Build history of the part. All positions in model axes, mm. Face numbers are marked on the shaded views. A direction names the side the tool comes from. Round coordinates to 2 decimals unless told otherwise and drop trailing zeros. Loops run counter-clockwise (first coordinate to the right, second up) from the corner with the lowest first, then second, coordinate; pieces in that order, holes last.
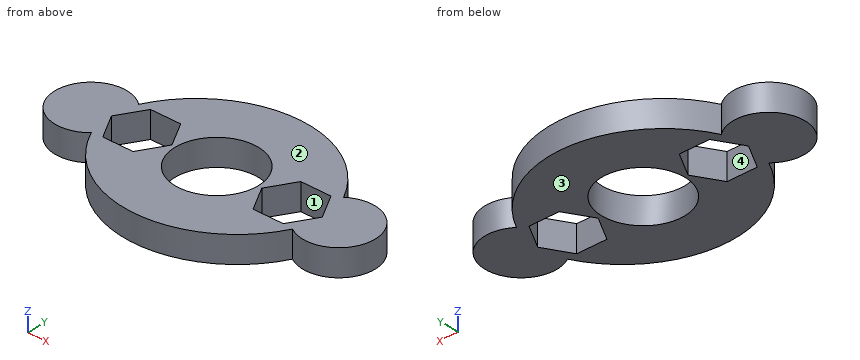
from build123d import *

# Parameters (mm, degrees)
F0_R     = 10.95
F1_DEPTH = 7


with BuildPart() as f1:
    # F0 (on Top) → F1 (new body)
    with BuildSketch(Plane.XY):
        with BuildLine():
            ThreePointArc((26.886002, -7.262236), (28.368444, -3.711389), (29.384189, 0))
            ThreePointArc((29.384189, 0), (28.162244, 4.291398), (26.317312, 8.35409))
            ThreePointArc((26.317312, 8.35409), (-0.849322, 23.940708), (-27.090225, 6.841477))
            ThreePointArc((-27.090225, 6.841477), (-28.443651, 3.48996), (-29.384189, 0))
            ThreePointArc((-29.384189, 0), (-28.351909, -3.759326), (-26.840855, -7.35305))
            ThreePointArc((-26.840855, -7.35305), (0.050708, -23.95269), (26.886002, -7.262236))
        make_face()
        Polygon((-28.139647, 0), (-24.098195, 7), (-16.015291, 7), (-11.973839, 0), (-16.015291, -7), (-24.098195, -7), align=None, mode=Mode.SUBTRACT)
        Circle(F0_R, mode=Mode.SUBTRACT)
        Polygon((28.21831, 0), (24.176858, -7), (16.093955, -7), (12.052503, 0), (16.093955, 7), (24.176858, 7), align=None, mode=Mode.SUBTRACT)
        with BuildLine():
            ThreePointArc((-29.384189, 0), (-28.443651, 3.48996), (-27.090225, 6.841477))
            ThreePointArc((-27.090225, 6.841477), (-42.77684, -0.53356), (-26.840855, -7.35305))
            ThreePointArc((-26.840855, -7.35305), (-28.351909, -3.759326), (-29.384189, 0))
        make_face()
        with BuildLine():
            ThreePointArc((26.317312, 8.35409), (28.162244, 4.291398), (29.384189, 0))
            ThreePointArc((29.384189, 0), (28.368444, -3.711389), (26.886002, -7.262236))
            ThreePointArc((26.886002, -7.262236), (41.495648, 1.088313), (26.317312, 8.35409))
        make_face()
    extrude(amount=F1_DEPTH)


solid = f1.part
(1) Pin check, flat tips, straight feed: P1, Ø4, axis at y = -10, z = 6, coming from the -X side; P2, Ø1.5, axis at y = 3, z = 2, coming from the -X side; P3, Ø1.5, axis at x = -13, z = 2.5, coming from the +Y side. Stop position of each tip, or through.
Responses:
P1: stops at x = -38.93
P2: stops at x = -42.41
P3: stops at y = 21.34
(2) Pull direction X, two halves, no side cores. Call the marked faces 1 and 2: +X half, -X half, draft (parallel to the pull), parting line (faces both ways), or undercut.
Responses:
face 1: undercut
face 2: draft
(3) Which spindle directions (+Z, -Z, +X, -X, +Y, -Y) get a long thin tool onto all of the face, cutting with end or side? Do the marked faces 3 and 4. Say none if no direction does.
Responses:
face 3: -Z, +X, -X, +Y, -Y
face 4: +Z, -Z
(4) Slice it at D-D on z = 2.25. List the corners of the cut face in (x, y), plus the area to 3 significant figures.
Responses:
outline: (-27.09, 6.84) arc R9.5 ccw (long way) to (-26.84, -7.35) arc R30 ccw to (26.89, -7.26) arc R9.5 ccw (long way) to (26.32, 8.35) arc R30 ccw to start; hole (-28.14, 0) - (-24.1, -7) - (-16.02, -7) - (-11.97, 0) - (-16.02, 7) - (-24.1, 7) - close; hole circle Ø21.9 at (0, 0); hole (12.05, 0) - (16.09, -7) - (24.18, -7) - (28.22, 0) - (24.18, 7) - (16.09, 7) - close
area: 1,840 mm2
(5) Slice it at B-B on y = -1.5. List the corners of the cut face in (x, z).
Responses:
outline: (-42.71, 0) - (-27.27, 0) - (-27.27, 7) - (-42.71, 7) - close; (-12.84, 0) - (-10.85, 0) - (-10.85, 7) - (-12.84, 7) - close; (10.85, 0) - (12.92, 0) - (12.92, 7) - (10.85, 7) - close; (27.35, 0) - (41.23, 0) - (41.23, 7) - (27.35, 7) - close
(6) Probe line 1 (Y direction, x = 0, z = 4.25); line 2 (Y direction, x = 0.5, z = 6); line 3 (X direction, y = -3.5, z = 3.5). List the from-to ranges inside material, lowest first.
Responses:
line 1: y = -23.95 to -10.95, 10.95 to 23.95
line 2: y = -23.95 to -10.94, 10.94 to 23.95
line 3: x = -42.25 to -26.12, -13.99 to -10.38, 10.38 to 14.07, 26.2 to 40.5
(7) Slice it at C-C on x = -19. List the corners of the cut face in (y, z).
Responses:
outline: (-17.17, 0) - (-7, 0) - (-7, 7) - (-17.17, 7) - close; (7, 0) - (17.17, 0) - (17.17, 7) - (7, 7) - close
(8) Slice it at A-A on x = 0. List the corners of the cut face in (y, z), plus the area to 3 significant figures.
Responses:
outline: (-23.95, 0) - (-10.95, 0) - (-10.95, 7) - (-23.95, 7) - close; (10.95, 0) - (23.95, 0) - (23.95, 7) - (10.95, 7) - close
area: 182 mm2
